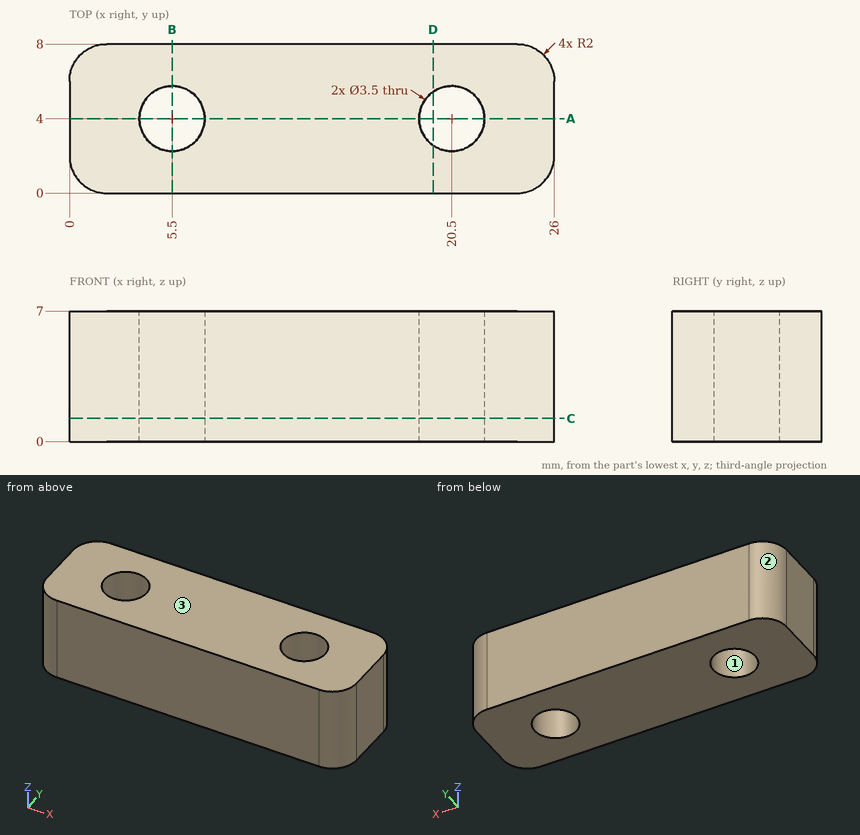
For this review, use the dimensioned drawing (mm, ordinates from the lowest corner) and the shaded views. Coordinates: 2 decimals unless noted, no trailing zeros. Write each loop counter-clockwise with the first axis right and the second up, starting at its lowest first coordinate (ties: lowest second). Pieces come first, ordered by that corner, then holes. Notation, with made-up numbers: (-18, 57.25) - (15, 57.25) arc R26 cw to (15, 92.25) - close; hole circle Ø7 at (79.25, 23.5). An arc over 180 degrees is marked (long way). Answer in a Markdown table with one row per item. Add a question column.
Q1. Draft analysis for pull direction Y (two halves, no side actions). For the marked faces 1, 2 and 3, state which applies: +Y half, -Y half, draft (parallel to the pull), parting line (faces both ways), or undercut.
Q2. Consider section B-B on x = 5.5. Give the boundary of the cut face in (y, z).
Q3. Consider section C-C on z = 1.25. Give the boundary of the cut face in (x, y), then the cut area to 3 significant figures.
Q4. Consider section D-D on x = 19.5. Give the boundary of the cut face in (y, z).
Q5. To check wall thickness, follow line 1 along X through (y, z) = (4, 1.5); line 2 along Y through (x, z) = (5.5, 2); line 3 along X through (y, z) = (5, 6.75). State the ranges of each line that lie inside material, in increasing order. Write a range as from..to.
Q6. Consider section A-A on y = 4. Give the boundary of the cut face in (x, z).
Answers below:
| question | item | result |
|---|---|---|
| 1 | face 1 | undercut |
| 1 | face 2 | +Y half |
| 1 | face 3 | draft |
| 2 | outline | (0, 0) - (2.25, 0) - (2.25, 7) - (0, 7) - close; (5.75, 0) - (8, 0) - (8, 7) - (5.75, 7) - close |
| 3 | outline | (0, 2) arc R2 ccw to (2, 0) - (24, 0) arc R2 ccw to (26, 2) - (26, 6) arc R2 ccw to (24, 8) - (2, 8) arc R2 ccw to (0, 6) - close; hole circle Ø3.5 at (5.5, 4); hole circle Ø3.5 at (20.5, 4) |
| 3 | area | 185 mm² |
| 4 | outline | (0, 0) - (2.56, 0) - (2.56, 7) - (0, 7) - close; (5.44, 0) - (8, 0) - (8, 7) - (5.44, 7) - close |
| 5 | line 1 | 0..3.75, 7.25..18.75, 22.25..26 |
| 5 | line 2 | 0..2.25, 5.75..8 |
| 5 | line 3 | 0..4.06, 6.94..19.06, 21.94..26 |
| 6 | outline | (0, 0) - (3.75, 0) - (3.75, 7) - (0, 7) - close; (7.25, 0) - (18.75, 0) - (18.75, 7) - (7.25, 7) - close; (22.25, 0) - (26, 0) - (26, 7) - (22.25, 7) - close |
